from build123d import *

# Parameters (mm, degrees)
SKETCH1_R           = 3.2
SKETCH1_R_2         = 1.25
BOSS_EXTRUDE1_DEPTH = 1.65
SKETCH2_W           = 32
SKETCH2_H           = 16
BOSS_EXTRUDE2_DEPTH = 6.2
SKETCH1_2_R         = 3.2
BOSS_EXTRUDE3_DEPTH = 2.65
SKETCH3_W           = 32.03
SKETCH3_H           = 10
BOSS_EXTRUDE4_DEPTH = 5.5


with BuildPart() as part:
    # Sketch1 → Boss-Extrude1 (new body)
    with BuildSketch(Plane.XY):
        with BuildLine():
            Line((-20, 18), (20, 18))
            ThreePointArc((20, 18), (22.121320344, 17.121320344), (23, 15))
            Line((23, 15), (23, -23))
            ThreePointArc((23, -23), (22.416236427, -24.864680631), (20.873373788, -26.063592072))
            Line((20.873373788, -26.063592072), (17.047054496, -27.491625922))
            ThreePointArc((17.047054496, -27.491625922), (16.287418762, -28.081915652), (16, -29))
            Line((16, -29), (16, -35))
            Line((16, -35), (-16, -35))
            Line((-16, -35), (-16, -29))
            ThreePointArc((-16, -29), (-16.287418762, -28.081915652), (-17.047054496, -27.491625922))
            Line((-17.047054496, -27.491625922), (-20.873373788, -26.063592072))
            ThreePointArc((-20.873373788, -26.063592072), (-22.416236427, -24.864680631), (-23, -23))
            Line((-23, -23), (-23, 15))
            ThreePointArc((-23, 15), (-22.121320344, 17.121320344), (-20, 18))
        make_face()
        Circle(SKETCH1_R, mode=Mode.SUBTRACT)
        with Locations((20, 15)):
            Circle(SKETCH1_R_2, mode=Mode.SUBTRACT)
        with Locations((-20, 15)):
            Circle(SKETCH1_R_2, mode=Mode.SUBTRACT)
        with Locations((-20, -23)):
            Circle(SKETCH1_R_2, mode=Mode.SUBTRACT)
        with Locations((20, -23)):
            Circle(SKETCH1_R_2, mode=Mode.SUBTRACT)
    extrude(amount=BOSS_EXTRUDE1_DEPTH)

    # Sketch2 → Boss-Extrude2 (add)
    with BuildSketch(Plane.XY.offset(1.65)):
        with Locations((0, -27)):
            Rectangle(SKETCH2_W, SKETCH2_H)
    extrude(amount=BOSS_EXTRUDE2_DEPTH)

    # Sketch1<2> → Boss-Extrude3 (add)
    with BuildSketch(Plane.XY):
        Circle(SKETCH1_2_R)
    extrude(amount=BOSS_EXTRUDE3_DEPTH)

    # Sketch3 → Boss-Extrude4 (add)
    with BuildSketch(Plane(origin=(0, 0, 0), x_dir=(-1, 0, 0), z_dir=(0, 0, -1))):
        with Locations((0.015, -30)):
            Rectangle(SKETCH3_W, SKETCH3_H)
    extrude(amount=BOSS_EXTRUDE4_DEPTH)


solid = part.part
Here's how the part is built. I have some questions about the finished solid (model axes, mm). A direction names the side the tool comes from. Coordinates: 2 decimals unless noted, no trailing zeros. Order: outer loops, then holes, each group sorted by start corner. A loop starts at its lowest first (then second) coordinate and runs counter-clockwise, first axis right, second up. Notation, with made-up numbers: M 21.5,-5 L 53.5,-5 A19 ccw 53.5,7 Z; hole C 46.5,45 d10. An arc over 180 degrees is marked long. Answer as CSV lines item,"result". Start each with the question number.
1. I want a section at D-D, the plane z = -2.5. Write out the boundary of the cut face in (x, y), and give its area (3 significant figures).
2. We'd pull the mould along Y, two halves only. Please class faces 4 (the cylindrical face through (20.672, 16.054, 0.813)), 5 (the cylindrical face through (22.1, 17.14, 0.81)), 6 (the flat face through (0, -35, 1)): released by +Y, released by -Y, zero draft, split by the parting line, or undercut.
3. For pin 1 (3 mm diameter, centred on x = -20, y = 15, fed in from +Z); pin 2 (2.5 mm diameter, centred on y = -29.5, z = 4, fed in from -X); pin 3 (4 mm diameter, centred on y = 9.5, z = 4, fed in from -X); pin 4 (7 mm diameter, centred on x = 1, y = 0, fed in from +Z), each with a flat end and sliding along its axis, tell me the tip position at first contact or that it passes through.
4. I want a section at A-A, the plane x = 0. Write out the boundary of the cut face in (y, z).
5. I need wall thicknesses on line 1 (Y direction, x = -20, z = 1.1); line 2 (Y direction, x = -14.5, z = -2); line 3 (Z direction, x = -5.5, y = -2). Which ranges of each line are inside material? Lowest first, please. Write a range as [from, to].
6. I want a section at C-C, the plane x = 12.5. Write out the boundary of the cut face in (y, z), and give its area (3 significant figures).
7. I want a section at B-B, the plane y = 0. Write out the boundary of the cut face in (x, z).
8. On a 3-axis mill with a long thin cutter (end or side, diameter ignored), from which of +Z, -Z, +X, -X, +Y, -Y can I reach the whole of each face in a straight line? I mean faces 1 (the cylindrical face through (-2.539, -1.947, 2.143)), 2 (the flat face through (-16.03, -30, -3)), 3 (the flat face through (0, 0, 2.65)). Say none if no direction works.
Recorded:
1,outline,"M -16.03,-35 L 16,-35 L 16,-25 L -16.03,-25 Z"
1,area,"320 mm2"
2,face 4,"undercut"
2,face 5,"released by +Y"
2,face 6,"released by -Y"
3,pin 1,"stops at z = 1.65"
3,pin 2,"stops at x = -16"
3,pin 3,"passes through"
3,pin 4,"stops at z = 2.65"
4,outline,"M -35,-5.5 L -25,-5.5 L -25,0 L 18,0 L 18,1.65 L 3.2,1.65 L 3.2,2.65 L -3.2,2.65 L -3.2,1.65 L -19,1.65 L -19,7.85 L -35,7.85 Z"
5,line 1,"y = [-26.39, -24.25], [-21.75, 13.75], [16.25, 18]"
5,line 2,"y = [-35, -25]"
5,line 3,"z = [0, 1.65]"
6,outline,"M -35,-5.5 L -25,-5.5 L -25,0 L 18,0 L 18,1.65 L -19,1.65 L -19,7.85 L -35,7.85 Z"
6,area,"242 mm2"
7,outline,"M -23,0 L 23,0 L 23,1.65 L 3.2,1.65 L 3.2,2.65 L -3.2,2.65 L -3.2,1.65 L -23,1.65 Z"
8,face 1,"+Z"
8,face 2,"-Z, -X, +Y, -Y"
8,face 3,"+Z, +X, -X, +Y"
